Part model, mm, in its own coordinate system. Face numbers are marked on the shaded views. A direction names the side the tool comes from. Give positions to 0.01 mm unless a question says otherwise; leave off trailing zeros. Write each loop counter-clockwise with the first axis right and the second up, starting at its lowest first coordinate (ties: lowest second). Pieces come first, ordered by that corner, then holes.
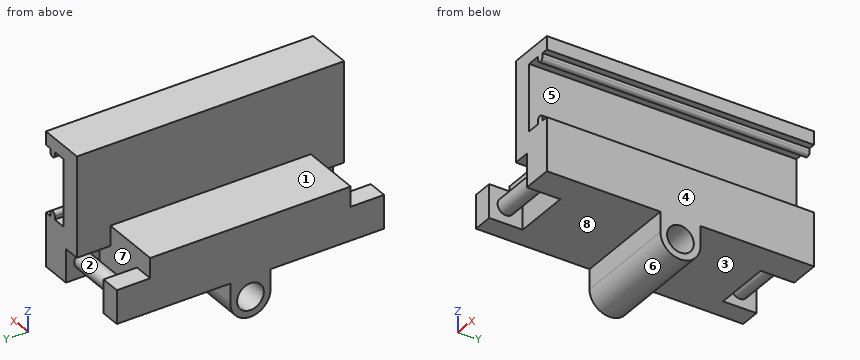
Autodesk Inventor part; units mm, degrees
ref_plane "YZ Plane" through (0, 0, 0) normal (1, 0, 0) x (0, 1, 0)
ref_plane "XZ Plane" through (0, 0, 0) normal (0, 1, 0) x (-1, 0, 0)
ref_plane "XY Plane" through (0, 0, 0) normal (0, 0, 1) x (1, 0, 0)
sketch "Sketch1" plane through (0, 0, 0) normal (0, 1, 0) x (-1, 0, 0)
  line L0 (0, 0) -> (0, 2)
  line L1 (0, 2) -> (7, 2)
  line L2 (7, 2) -> (7, -18)
  line L3 (7, -18) -> (0, -18)
  line L4 (0, -18) -> (0, -10)
  line L5 (0, -10) -> (4, -10)
  line L6 (4, -10) -> (4, 0)
  line L7 (4, 0) -> (0, 0)
  dimension "d0" = 2
  dimension "d1" = 7
  dimension "d2" = 20
  dimension "d3" = 7
  dimension "d4" = 8
  dimension "d5" = 4
  dimension "d6" = 10
extrude "Extrusion1" add sketch "Sketch1" along normal blind 40
sketch "Sketch5" plane through (0, 0, 0) normal (0, -1, 0) x (1, 0, 0)
  line L0 (-1, -10) -> (-1, -9.5)
  line L1 (-1.5, -9) -> (-1.5, -9)
  line L2 (-2, -9.5) -> (-2, -10)
  line L3 (-2, -10) -> (-1, -10)
  line L4 (-1, -0.5) -> (-1, 0)
  line L5 (-1, 0) -> (-2, 0)
  line L6 (-2, 0) -> (-2, -0.5)
  line L7 (-1.5, -1) -> (-1.5, -1)
  arc A0 (-1.5, -9) -> (-2, -9.5) centre (-1.5, -9.5) ccw
  arc A1 (-1, -9.5) -> (-1.5, -9) centre (-1.5, -9.5) ccw
  arc A2 (-2, -0.5) -> (-1.5, -1) centre (-1.5, -0.5) ccw
  arc A3 (-1.5, -1) -> (-1, -0.5) centre (-1.5, -0.5) ccw
  point P0 (0, 0)
  point P1 (-1, -9)
  point P2 (-2, -9)
  point P3 (-1, -1)
  point P4 (-2, -1)
  point P5 (-1.5, 0)
  point P6 (-1.5, -10)
  point P7 (0, -10)
  dimension "d35" = 1
  dimension "d36" = 1
  dimension "d37" = 1
  dimension "d38" = 1
  dimension "d39" = 1
  dimension "d40" = 1
  dimension "d41" = 0.5
  dimension "d42" = 1
  dimension "d43" = 1
extrude "Extrusion2" add sketch "Sketch5" against normal blind 40
sketch "Sketch7" plane through (-7, 0, -18) normal (-1, 0, 0) x (0, 0, 1)
  line L0 (8, 0) -> (8, 5)
  line L1 (8, 0) -> (8, 40)
  line L2 (8, 5) -> (0, 5)
  line L3 (0, 0) -> (0, 40)
  line L4 (0, 35) -> (8, 35)
  line L5 (8, 40) -> (8, 0)
  line L6 (0, 0) -> (8, 0)
  point P0 (18, 0)
  dimension "d51" = 5
extrude "Extrusion4" add sketch "Sketch7" along normal blind 9
sketch "Sketch8" plane through (-16, 0, -18) normal (-1, 0, 0) x (0, 0, 1)
  line L0 (0, 40) -> (20, 40)
  line L1 (20, 0) -> (8, 0)
  line L2 (0, 40) -> (0, 23)
  line L3 (0, 0) -> (0, 40)
  line L4 (0, 23) -> (-3, 23)
  line L5 (0, 0) -> (0, 17)
  line L6 (0, 17) -> (-3, 17)
  arc A0 (-3, 23) -> (-3, 17) centre (-3, 20) ccw
  circle A1 centre (-3, 20) radius 2
  point P0 (18, 0)
  dimension "d56" = 40
  dimension "d57" = 17
  dimension "d58" = 3
  dimension "d59" = 17
  dimension "d60" = 3
  dimension "d61" = 4
extrude "Extrusion5" add sketch "Sketch8" against normal blind 16
sketch "Sketch10" plane through (-7, 0, -18) normal (-1, 0, 0) x (0, 0, 1)
  line L0 (0, 0) -> (5, 0)
  line L1 (5, 0) -> (5, 5)
  line L2 (5, 5) -> (0, 5)
  line L3 (0, 5) -> (0, 0)
  line L4 (0, 35) -> (5, 35)
  line L5 (5, 35) -> (5, 40)
  line L6 (5, 40) -> (0, 40)
  line L7 (0, 40) -> (0, 35)
  point P0 (18, 0)
  dimension "d64" = 5
  dimension "d65" = 5
  dimension "d66" = 5
  dimension "d67" = 5
extrude "Extrusion6" cut sketch "Sketch10" against normal blind 2.5
sketch "Sketch11" plane through (-16, 0, -18) normal (-1, 0, 0) x (0, 0, 1)
  line L0 (0, 0) -> (8, 0)
  line L1 (8, 0) -> (8, 5)
  line L2 (8, 5) -> (0, 5)
  line L3 (0, 5) -> (0, 0)
  point P0 (18, 0)
  dimension "d70" = 8
  dimension "d71" = 5
extrude "Extrusion7" cut sketch "Sketch11" against normal blind 9
sketch "Sketch12" plane through (-4.5, 0, -18) normal (-1, 0, 0) x (0, 0, 1)
  circle A0 centre (2.5, 2.5) radius 1.25
  circle A1 centre (2.5, 37.5) radius 1.25
  point P0 (18, 0)
  dimension "d74" = 2.5
  dimension "d75" = 2.5
extrude "Extrusion8" add sketch "Sketch12" along normal blind 11.5
sketch "Sketch14" plane through (-16, 0, -18) normal (-1, 0, 0) x (0, 0, 1)
  line L0 (0, 35) -> (5, 35)
  line L1 (5, 40) -> (5, 35)
  line L2 (5, 35) -> (5, 40)
  line L3 (5, 40) -> (0, 40)
  line L4 (8, 40) -> (0, 40)
  line L5 (0, 40) -> (0, 35)
  line L6 (0, 23) -> (0, 40)
  line L7 (0, 5) -> (0, 0)
  line L8 (0, 0) -> (5, 0)
  line L9 (5, 0) -> (5, 5)
  line L10 (0, 5) -> (8, 5)
  line L11 (5, 5) -> (0, 5)
  line L12 (0, 5) -> (5, 5)
  point P0 (18, 0)
extrude "Extrusion9" add sketch "Sketch14" against normal blind 3
sketch "Sketch4" plane through (-4, 0, 0) normal (1, 0, 0) x (0, 0, -1)
  point P0 (5, 30)
  point P1 (5, 10)
properties part number "Karetka"
1) Saw through at B-B, the plane z = -15.5. Write the cut outline in (x, y), then the cut area to 4 significant figures.
Answers follow:
outline: (-16, 0) - (-13, 0) - (-13, 1.25) - (-4.5, 1.25) - (-4.5, 0) - (0, 0) - (0, 40) - (-4.5, 40) - (-4.5, 38.75) - (-13, 38.75) - (-13, 40) - (-16, 40) - close; hole (-13, 3.75) - (-4.5, 3.75) - (-4.5, 5) - (-13, 5) - close; hole (-13, 35) - (-4.5, 35) - (-4.5, 36.25) - (-13, 36.25) - close
area: 597.5 mm2
2) Two-plate mould, pull along Y, no slides. Class the marked faces 6, 7 and 8: +Y half, -Y half, draft (parallel to the pull), parting line (faces both ways), or undercut.
Answers follow:
face 6: parting line
face 7: undercut
face 8: draft
3) Saw through at C-C, the plane y = 2.5. Write the cut outline in (x, z), then the cut area to 3 significant figures.
Answers follow:
outline: (-16, -18) - (-13, -18) - (-13, -16.75) - (-4.5, -16.75) - (-4.5, -18) - (0, -18) - (0, -10) - (-1, -10) - (-1, -9.5) arc R0.5 ccw to (-2, -9.5) - (-2, -10) - (-4, -10) - (-4, 0) - (-2, 0) - (-2, -0.5) arc R0.5 ccw to (-1, -0.5) - (-1, 0) - (0, 0) - (0, 2) - (-7, 2) - (-7, -13) - (-4.5, -13) - (-4.5, -14.25) - (-13, -14.25) - (-13, -13) - (-16, -13) - close
area: 126 mm2
4) Saw through at D-D, the plane z = -11.25. Write the cut outline in (x, y), then the cut area to 3 significant figures.
Answers follow:
outline: (-16, 5) - (-7, 5) - (-7, 0) - (0, 0) - (0, 40) - (-7, 40) - (-7, 35) - (-16, 35) - close
area: 550 mm2
5) Pin check, flat tips, straight feed: pin 1 Ø1.5 at (x, z) = (-5.5, -20) entering from -Y; pin 2 Ø2 at (x, y) = (-6, 3) entering from -Z; pin 3 Ø8 at (x, y) = (-9, 33.5) entering from -Z; pin 4 Ø1.5 at (y, z) = (12, -20) entering from -X. Stop position of each tip, or through.
Answers follow:
pin 1: stops at y = 17
pin 2: stops at z = -16.75
pin 3: stops at z = -18
pin 4: passes through
6) Saw through at A-A, the plane x = -1.5. Write the cut outline in (y, z), then the cut area to 3 significant figures.
Answers follow:
outline: (0, -18) - (17, -18) - (17, -21) arc R3 ccw to (23, -21) - (23, -18) - (40, -18) - (40, -9) - (0, -9) - close; (0, -1) - (40, -1) - (40, 2) - (0, 2) - close; hole circle Ø4 at (20, -21)
area: 500 mm2
7) Wall check: L1, parallel to Y at x = -11, z = -21; L2, parallel to Z at x = -3.5, y = 32; L3, parallel to X at y = 3, z = -0.25. Give the ranges that are in metal, low to high.
Answers follow:
L1: y = 17 to 18, 22 to 23
L2: z = -18 to -10, 0 to 2
L3: x = -7 to -4, -2 to -1
8) 3-axis set-ups, long thin cutter, end or side, ignore diameter. For the marked faces 1, 2, 3, 4 and 5: which of +Z, -Z, +X, -X, +Y, -Y reach the whole face in a straight line?
Answers follow:
face 1: +Z, -X, +Y, -Y
face 2: none
face 3: -Z, +X, -X, +Y
face 4: +Z, -Z, +X, +Y, -Y
face 5: +Y, -Y
